Geometry: see drawing. Coordinates: mm, zero at the bounding-box minimum. Round coordinates to 2 decimals unless told otherwise and drop trailing zeros. Loops run counter-clockwise (first coordinate to the right, second up) from the corner with the lowest first, then second, coordinate; pieces in that order, holes last. Notation, with made-up numbers: (23.5, 1.25) -> (50.5, 1.25) arc R25 cw to (50.5, 36.25) -> close; hole circle Ø11 at (62.25, 34). An arc over 180 degrees is marked (long way). Answer in a Markdown table with one row per item.
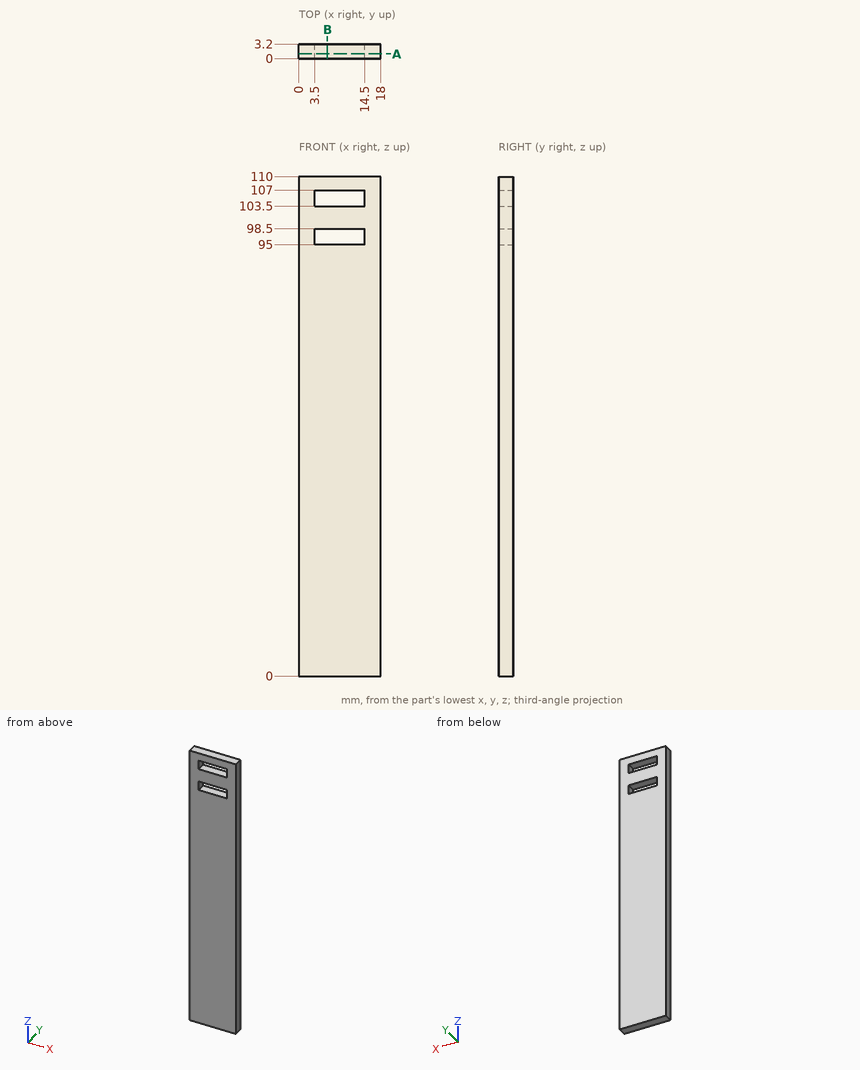
Item 1: Section query A-A, the plane y = 1.05. Output: boundary loops of the cut face in (x, z), and give its area (3 significant figures).
Ans:
| item | result |
|---|---|
| outline | (0, 0) -> (18, 0) -> (18, 110) -> (0, 110) -> close; hole (3.5, 95) -> (14.5, 95) -> (14.5, 98.5) -> (3.5, 98.5) -> close; hole (3.5, 103.5) -> (14.5, 103.5) -> (14.5, 107) -> (3.5, 107) -> close |
| area | 1,900 mm2 |
Item 2: Ray query, L1, parallel to Z at x = 8, y = 1.9. Return the intervals inside material, ascending.
Ans:
| item | result |
|---|---|
| L1 | 0 to 95, 98.5 to 103.5, 107 to 110 |
Item 3: Section query B-B, the plane x = 6.25. Output: boundary loops of the cut face in (y, z), and give its area (3 significant figures).
Ans:
| item | result |
|---|---|
| outline | (0, 0) -> (3.2, 0) -> (3.2, 95) -> (0, 95) -> close; (0, 98.5) -> (3.2, 98.5) -> (3.2, 103.5) -> (0, 103.5) -> close; (0, 107) -> (3.2, 107) -> (3.2, 110) -> (0, 110) -> close |
| area | 330 mm2 |
